Autodesk Inventor part; units mm, degrees
ref_plane "YZ Plane" through (0, 0, 0) normal (1, 0, 0) x (0, 1, 0)
ref_plane "XZ Plane" through (0, 0, 0) normal (0, 1, 0) x (-1, 0, 0)
ref_plane "XY Plane" through (0, 0, 0) normal (0, 0, 1) x (1, 0, 0)
sketch "Sketch1" plane through (0, 0, 0) normal (0, 0, 1) x (1, 0, 0)
  circle A0 centre (0, 0) radius 96.5685 construction
  circle A1 centre (0, 0) radius 140 construction
  line L0 (140, -140) -> (-140, -140)
  line L1 (-140, -140) -> (-140, 140)
  line L2 (-140, 140) -> (140, 140)
  line L3 (140, 140) -> (140, -140)
  line L4 (140, -140) -> (-140, 140) construction
  line L5 (-140, -140) -> (140, 140) construction
  line L6 (57.9899, 140) -> (140, 57.9899)
  line L7 (140, 57.9899) -> (140, -57.9899)
  line L8 (140, -57.9899) -> (57.9899, -140)
  line L9 (57.9899, -140) -> (-57.9899, -140)
  line L10 (-57.9899, -140) -> (-140, -57.9899)
  line L11 (-140, -57.9899) -> (-140, 57.9899)
  line L12 (-140, 57.9899) -> (-57.9899, 140)
  line L13 (-57.9899, 140) -> (57.9899, 140)
  line L14 (40, 96.5685) -> (96.5685, 40)
  line L15 (96.5685, 40) -> (96.5685, -40)
  line L16 (96.5685, -40) -> (40, -96.5685)
  line L17 (40, -96.5685) -> (-40, -96.5685)
  line L18 (-40, -96.5685) -> (-96.5685, -40)
  line L19 (-96.5685, -40) -> (-96.5685, 40)
  line L20 (-96.5685, 40) -> (-40, 96.5685)
  line L21 (-40, 96.5685) -> (40, 96.5685)
  point P0 (0, 140)
  point P1 (-57.9899, 140)
  point P2 (-140, 57.9899)
  point P3 (-140, -57.9899)
  point P4 (-57.9899, -140)
  point P5 (57.9899, -140)
  point P6 (140, -57.9899)
  point P7 (140, 57.9899)
  point P8 (57.9899, 140)
  point P9 (0, 96.5685)
  point P10 (0, 140)
  dimension "d23" = 280
  dimension "d41" = 80
  dimension "d42" = 43.4315
extrude "Plate1" add sketch "Sketch1" along normal blind 4 contours L0 L10 L1 L12 L2 L6 L3 L8
sketch "Sketch6" plane through (0, 0, 0) normal (0, 0, 1) x (1, 0, 0)
  line L0 (0, 0) -> (0, 120) construction
  circle A0 centre (0, 0) radius 120 construction
  line L1 (0, 0) -> (84.8528, 84.8528) construction
  circle A1 centre (84.8528, 84.8528) radius 9
  dimension "d32" = 18
  dimension "d33" = 240
  dimension "d34" = 45
extrude "Cut2" cut sketch "Sketch6" along normal blind 4
pattern_circular "Circular Pattern2" count 3 over 90 about axis through (0, 0, -10) along (0, 0, -1) of "Cut2"
mirror "Mirror1" about plane through (0, 0, 0) normal (1, 0, 0) of "Cut2", "Circular Pattern2"
equation "\"d23\" = Flange_D_outer"
equation "\"d32\" = Flange_d_hole_diam"
equation "\"d33\" = Flange_D1_hole_center"
equation "\"d35\" = Thickness"
equation "\"d2\" = Thickness"
equation "\"BendReliefWidth\" = Thickness"
equation "\"BendReliefDepth\" = 0.5 * Thickness"
equation "\"CornerReliefSize\" = 4 * Thickness"
equation "\"MinimumRemnant\" = 2 * Thickness"
equation "\"TransitionRadius\" = BendRadius"
equation "\"JacobiRadiusSize\" = BendRadius"
equation "\"GapSize\" = Thickness"
equation "\"Octaeder_flange_lenth\" = d42"
properties part number "DSB 110 drain sustem flange" material "Stainless Steel"
Could you check a few things on this model? Use its own coordinates, in mm. A direction names the side the tool comes from. Round coordinates to 2 decimals unless told otherwise and drop trailing zeros. Loops run counter-clockwise (first coordinate to the right, second up) from the corner with the lowest first, then second, coordinate; pieces in that order, holes last.
Q1. I want a section at D-D (y = 88.5). Write out the boundary of the cut face in (x, z).
Q2. Thinking about a two-plate mould opening in X: for faces 1 (the flat face through (99.57, -98.42, 1.97)), 2 (the flat face through (67.89, 68.68, 1.97)), 3 (the cylindrical face through (89.691, 77.264, 1.972)), 4 (the flat face through (-95, 64, 0)), which applies, pulls with the +X half, pulls with the -X half, needs draft (parallel to the pull), parting line crosses it, or undercut?
Q3. I want a section at A-A (x = 3). Write out the boundary of the cut face in (y, z).
Q4. Please list where these lines run through material, in increasing order: L1, parallel to X at y = 0, z = 1.9; L2, parallel to X at y = -1, z = 1.65; L3, parallel to Y at x = 5, z = 2.75.
Q5. On a 3-axis mill with a long thin cutter (end or side, diameter ignored), from which of +Z, -Z, +X, -X, +Y, -Y can I reach the whole of each face in a straight line? I mean faces 5 (the flat face through (-67.89, -68.68, 1.97)), 6 (the flat face through (-95, 64, 4)). Say none if no direction works.
Q6. I want a section at B-B (y = 0). Write out the boundary of the cut face in (x, z).
Q7. For P1, Ø1.5, axis at y = -94, z = 2, coming from the -X side; P2, Ø11, axis at x = 120, y = 0, coming from the +Z side; P3, Ø1, axis at y = -82.5, z = 3.5, coming from the -X side, each with a flat end and sliding along its axis, tell me the tip position at first contact or that it passes through.
Q8. I want a section at C-C (z = 0.7). Write out the boundary of the cut face in (x, y).
Answer below:
1. outline: (-109.49, 0) - (-93.08, 0) - (-93.08, 4) - (-109.49, 4) - close; (-76.62, 0) - (-48.07, 0) - (-48.07, 4) - (-76.62, 4) - close; (48.07, 0) - (76.62, 0) - (76.62, 4) - (48.07, 4) - close; (93.08, 0) - (109.49, 0) - (109.49, 4) - (93.08, 4) - close
2. face 1: pulls with the +X half
2. face 2: undercut
2. face 3: undercut
2. face 4: needs draft
3. outline: (-140, 0) - (-96.57, 0) - (-96.57, 4) - (-140, 4) - close; (96.57, 0) - (140, 0) - (140, 4) - (96.57, 4) - close
4. L1: x = -140 to -129, -111 to -96.57, 96.57 to 111, 129 to 140
4. L2: x = -140 to -128.94, -111.06 to -96.57, 96.57 to 111.06, 128.94 to 140
4. L3: y = -140 to -96.57, 96.57 to 140
5. face 5: +Z, -Z
5. face 6: +Z, +X, -X, +Y, -Y
6. outline: (-140, 0) - (-129, 0) - (-129, 4) - (-140, 4) - close; (-111, 0) - (-96.57, 0) - (-96.57, 4) - (-111, 4) - close; (96.57, 0) - (111, 0) - (111, 4) - (96.57, 4) - close; (129, 0) - (140, 0) - (140, 4) - (129, 4) - close
7. P1: stops at x = -104.74
7. P2: passes through
7. P3: stops at x = -115.99
8. outline: (-140, -57.99) - (-57.99, -140) - (57.99, -140) - (140, -57.99) - (140, 57.99) - (57.99, 140) - (-57.99, 140) - (-140, 57.99) - close; hole circle Ø18 at (-120, 0); hole (-96.57, -40) - (-40, -96.57) - (40, -96.57) - (96.57, -40) - (96.57, 40) - (40, 96.57) - (-40, 96.57) - (-96.57, 40) - close; hole circle Ø18 at (-84.85, -84.85); hole circle Ø18 at (-84.85, 84.85); hole circle Ø18 at (84.85, -84.85); hole circle Ø18 at (84.85, 84.85); hole circle Ø18 at (120, 0)
